The listing builds one solid part. Answer for the finished solid, in the listing's coordinates (mm). Face numbers are marked on the shaded views. A direction names the side the tool comes from. Round coordinates to 2 decimals unless told otherwise and drop trailing zeros. Write each loop counter-clockwise with the first axis right and the second up, starting at its lowest first coordinate (ties: lowest second). Pieces come first, ordered by that corner, then holes. Notation, with made-up numbers: (23, -4.75) - (60, -4.75) arc R22 ccw to (60, 15.25) - close; hole circle Ø8 at (87, 27). An arc over 180 degrees is marked (long way). Use a Markdown table: item, result. Add a question column.
1) A tool of negligible diameter and unlimited length cuts with its end or side. For the marked faces 1 and 2, from which of +Z, -Z, +X, -X, +Y, -Y can it reach the whole face along a straight path? Write none if from no direction.
2) This flat-tipped pin is pushed along its axis until it touches: P1, Ø1.4, axis at x = 36.195, z = 25.4, coming from the +Y side. Where does it stop, or does it pass through?
3) A cutting plane is placed at C-C (y = 20.75). Give the vertices of the cut face in (x, z), then the cut area to 3 significant figures.
4) Determine the mould class of the marked faces 3, 4 and 5 for opening direction X: +X half, -X half, draft (parallel to the pull), parting line (faces both ways), or undercut.
5) A cutting plane is placed at B-B (z = 14). Give the vertices of the cut face in (x, y).
6) Find the intervals of material crossed by probe 1 along X at (y, z) = (20.25, 9); probe 2 along Z at (x, y) = (47.5, 12.7); probe 3 along Y at (x, z) = (8, 26), in increasing order. Write a range as from..to.
7) A cutting plane is placed at A-A (y = 12.7). Give the vertices of the cut face in (x, z), then the cut area to 3 significant figures.
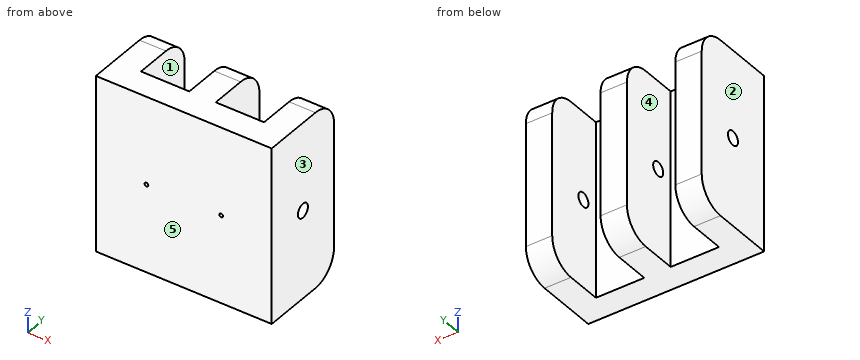
```python
from build123d import *

# Parameters (mm, degrees)
BOSS_EXTRUDE1_DEPTH = 50.8
FILLET3_R           = 7.62
FILLET4_R           = 7.62
SKETCH3_R           = 0.5334
CUT_EXTRUDE1_DEPTH  = 75.009515604
SKETCH4_R           = 2.032
CUT_EXTRUDE2_DEPTH  = 77.2


with BuildPart() as part:
    # 3DSketch1 → Boss-Extrude1 (new body)
    with BuildSketch(Plane(origin=(0, 25.4, 0), x_dir=(0.894427190999916, -0.447213595499958, 0), z_dir=(0, 0, -1))):
        Polygon((0, 0), (11.359225326, 22.718450651), (56.796126628, 0), (45.436901303, -22.718450651), (38.621366107, -19.310683054), (46.572823835, -3.407767598), (34.077675977, 2.839806331), (26.126218249, -13.063109125), (19.310683054, -9.655341527), (27.262140782, 6.247573929), (14.766992923, 12.495147858), (6.815535195, -3.407767598), align=None)
    extrude(amount=-BOSS_EXTRUDE1_DEPTH)

    # Fillet3
    fillet3_edges = [part.edges().sort_by_distance(p)[0] for p in [
        (3.81, 25.4, 50.8),
        (25.4, 25.4, 50.8),
        (46.99, 25.4, 50.8),
    ]]
    fillet(fillet3_edges, radius=FILLET3_R)

    # Fillet4
    fillet4_edges = [part.edges().sort_by_distance(p)[0] for p in [
        (46.99, 25.4, 0),
        (25.4, 25.4, 0),
        (3.81, 25.4, 0),
    ]]
    fillet(fillet4_edges, radius=FILLET4_R)

    # Sketch3 → Cut-Extrude1 (cut, through all)
    with BuildSketch(Plane(origin=(0, 7.62, 0), x_dir=(1, 0, 0), z_dir=(0, 1, 0))):
        with Locations(Location((14.605, -25.4, 0), (0, 0, 180))):
            Circle(SKETCH3_R)
        with Locations(Location((36.195, -25.4, 0), (0, 0, 180))):
            Circle(SKETCH3_R)
    extrude(amount=-CUT_EXTRUDE1_DEPTH, mode=Mode.SUBTRACT)

    # Sketch4 → Cut-Extrude2 (cut, through all)
    with BuildSketch(Plane(origin=(50.8, 0, 0), x_dir=(0, 0, -1), z_dir=(1, 0, 0))):
        with Locations(Location((-25.4, 12.7, 0), (0, 0, 90))):
            Circle(SKETCH4_R)
    extrude(amount=-CUT_EXTRUDE2_DEPTH, mode=Mode.SUBTRACT)


solid = part.part
```
Entries:
| question | item | result |
|---|---|---|
| 1 | face 1 | +Z, -Z, +Y |
| 1 | face 2 | +Z, -Z, -X, +Y, -Y |
| 2 | P1 | stops at y = 7.62 |
| 3 | outline | (0, 0.6) - (7.62, 0.6) - (7.62, 50.2) - (0, 50.2) - close; (21.59, 0.6) - (29.21, 0.6) - (29.21, 50.2) - (21.59, 50.2) - close; (43.18, 0.6) - (50.8, 0.6) - (50.8, 50.2) - (43.18, 50.2) - close |
| 3 | area | 1,130 mm² |
| 4 | face 3 | +X half |
| 4 | face 4 | undercut |
| 4 | face 5 | draft |
| 5 | outline | (0, 0) - (50.8, 0) - (50.8, 25.4) - (43.18, 25.4) - (43.18, 7.62) - (29.21, 7.62) - (29.21, 25.4) - (21.59, 25.4) - (21.59, 7.62) - (7.62, 7.62) - (7.62, 25.4) - (0, 25.4) - close |
| 6 | probe 1 | x = 0..7.62, 21.59..29.21, 43.18..50.8 |
| 6 | probe 2 | z = 0..23.37, 27.43..50.8 |
| 6 | probe 3 | y = 0..7.62 |
| 7 | outline | (0, 0) - (7.62, 0) - (7.62, 23.37) - (0, 23.37) - close; (0, 27.43) - (7.62, 27.43) - (7.62, 50.8) - (0, 50.8) - close; (21.59, 0) - (29.21, 0) - (29.21, 23.37) - (21.59, 23.37) - close; (21.59, 27.43) - (29.21, 27.43) - (29.21, 50.8) - (21.59, 50.8) - close; (43.18, 0) - (50.8, 0) - (50.8, 23.37) - (43.18, 23.37) - close; (43.18, 27.43) - (50.8, 27.43) - (50.8, 50.8) - (43.18, 50.8) - close |
| 7 | area | 1,070 mm² |
